For this review, take the finished solid that the model builds, in its own axes (mm). A direction names the side the tool comes from. Give positions to 0.01 mm unless a question says otherwise; leave off trailing zeros. Loops run counter-clockwise (first coordinate to the right, second up) from the corner with the lowest first, then second, coordinate; pieces in that order, holes last.
```python
from build123d import *

# Parameters (mm, degrees)
SKETCH1_W           = 60
SKETCH1_H           = 43
BOSS_EXTRUDE1_DEPTH = 25
SKETCH2_W           = 34
SKETCH2_H           = 25.5
BOSS_EXTRUDE2_DEPTH = 5
SKETCH5_W           = 34.00729927
SKETCH5_H           = 30
BOSS_EXTRUDE3_DEPTH = 10.5
SKETCH6_R           = 6
CUT_EXTRUDE1_DEPTH  = 86.803554705
SKETCH7_R           = 8.437552617
SKETCH7_R_2         = 5.978835127
CUT_EXTRUDE2_DEPTH  = 2.5


with BuildPart() as part:
    # Sketch1 → Boss-Extrude1 (new body)
    with BuildSketch(Plane(origin=(0, 0, 0), x_dir=(1, 0, 0), z_dir=(0, 1, 0))):
        with Locations((30, 21.5)):
            Rectangle(SKETCH1_W, SKETCH1_H)
    extrude(amount=BOSS_EXTRUDE1_DEPTH)

    # Sketch2 → Boss-Extrude2 (add)
    with BuildSketch(Plane(origin=(0, 25, 0), x_dir=(1, 0, 0), z_dir=(0, 1, 0))):
        with Locations((30, 30.25)):
            Rectangle(SKETCH2_W, SKETCH2_H)
    extrude(amount=BOSS_EXTRUDE2_DEPTH)

    # Sketch5 → Boss-Extrude3 (add)
    with BuildSketch(Plane(origin=(0, 0, -43), x_dir=(-1, 0, 0), z_dir=(0, 0, -1))):
        with Locations((-29.996350365, 15)):
            Rectangle(SKETCH5_W, SKETCH5_H)
    extrude(amount=BOSS_EXTRUDE3_DEPTH)

    # Sketch6 → Cut-Extrude1 (cut, through all)
    with BuildSketch(Plane(origin=(0, 30, 0), x_dir=(1, 0, 0), z_dir=(0, 1, 0))):
        with Locations(Location((29.998211201, 35.144717579, 0), (0, 0, 270))):
            Circle(SKETCH6_R)
    extrude(amount=-CUT_EXTRUDE1_DEPTH, mode=Mode.SUBTRACT)

    # Sketch7 → Cut-Extrude2 (cut, symmetric)
    with BuildSketch(Plane(origin=(0, 30, 0), x_dir=(1, 0, 0), z_dir=(0, 1, 0))):
        with Locations(Location((29.998209055, 35.165882453, 0), (0, 0, 270))):
            Circle(SKETCH7_R)
        with Locations((29.998209055, 35.165882453)):
            Circle(SKETCH7_R_2, mode=Mode.SUBTRACT)
    extrude(amount=CUT_EXTRUDE2_DEPTH, both=True, mode=Mode.SUBTRACT)


solid = part.part
```
Item 1: Take a section at B-B on z = -34. Give the boundary of the cut face in (x, y).
Answer:
outline: (0, 0) - (24.11, 0) - (24.11, 27.5) - (21.64, 27.5) - (21.64, 30) - (13, 30) - (13, 25) - (0, 25) - close; (35.89, 0) - (60, 0) - (60, 25) - (47, 25) - (47, 30) - (38.35, 30) - (38.35, 27.5) - (35.89, 27.5) - close
Item 2: For L1, parallel to Y at x = 33.5, z = -28; L2, parallel to Z at x = 55, y = 23; L3, parallel to Y at x = 3.5, z = -12, list the stretches that pass through material, from the lowest coordinate up.
Answer:
L1: y = 0 to 27.5
L2: z = -43 to 0
L3: y = 0 to 25
Item 3: Take a section at D-D on x = 45.5. Give the boundary of the cut face in (y, z), and give its area (3 significant figures).
Answer:
outline: (0, -53.5) - (30, -53.5) - (30, -17.5) - (25, -17.5) - (25, 0) - (0, 0) - close
area: 1,520 mm2
Item 4: Take a section at C-C on y = 8.5. Give the boundary of the cut face in (x, z).
Answer:
outline: (0, -43) - (12.99, -43) - (12.99, -53.5) - (47, -53.5) - (47, -43) - (60, -43) - (60, 0) - (0, 0) - close; hole circle Ø12 at (30, -35.14)
Item 5: The part is to be moulded in two halves that separate along Z. For faces 6 (the flat face through (28, 27.5, -41)), 7 (the flat face through (30, 15, -53.5)), 8 (the flat face through (30, 12, 0)), 9 (the flat face through (0, 12, -21)), say which applies: released by +Z, released by -Z, zero draft, split by the parting line, or undercut.
Answer:
face 6: undercut
face 7: released by -Z
face 8: released by +Z
face 9: zero draft
Item 6: Take a section at A-A on x = 28. Give the boundary of the cut face in (y, z), and give its area (3 significant figures).
Answer:
outline: (0, -53.5) - (30, -53.5) - (30, -43.36) - (27.5, -43.36) - (27.5, -40.8) - (0, -40.8) - close; (0, -29.49) - (27.5, -29.49) - (27.5, -26.97) - (30, -26.97) - (30, -17.5) - (25, -17.5) - (25, 0) - (0, 0) - close
area: 1,170 mm2
Item 7: Tool access review of faces 1 (the flat face through (53, 12, -43)), 2 (the flat face through (12.993, 15, -48)), 3 (the cylindrical face through (24.86, 28.77, -41.86)), 4 (the flat face through (30, 27, -17.5)), 5 (the flat face through (13, 27, -30)): name each direction out of +Z, -Z, +X, -X, +Y, -Y from which nothing blocks a thin tool from reaching the whole face with its end or side.
Answer:
face 1: -Z, +X, +Y, -Y
face 2: -Z, -X, +Y, -Y
face 3: +Y
face 4: +Z, +X, -X, +Y
face 5: +Z, -Z, -X, +Y
Item 8: Clearance check with flat-ended pins moving along their axes: pin 1 Ø2.5 at (y, z) = (28, -33.5) entering from -X; pin 2 Ø6.5 at (x, y) = (50.5, 13) entering from -Z; pin 3 Ø1.5 at (x, y) = (27.5, 28.5) entering from +Z. State where each tip first meets the part, or that it passes through.
Answer:
pin 1: stops at x = 13
pin 2: stops at z = -43
pin 3: stops at z = -17.5
